Geometry: final body of the model. Coordinates: model frame, mm. Round coordinates to 2 decimals unless told otherwise and drop trailing zeros. Order: outer loops, then holes, each group sorted by start corner. A loop starts at its lowest first (then second) coordinate and runs counter-clockwise, first axis right, second up. Notation, with made-up numbers: (48, 39) -> (83, 39) arc R35 cw to (83, 78) -> close; hole circle Ø7 at (85, 47). An arc over 180 degrees is marked (long way). Put each result on its own line as item: value.
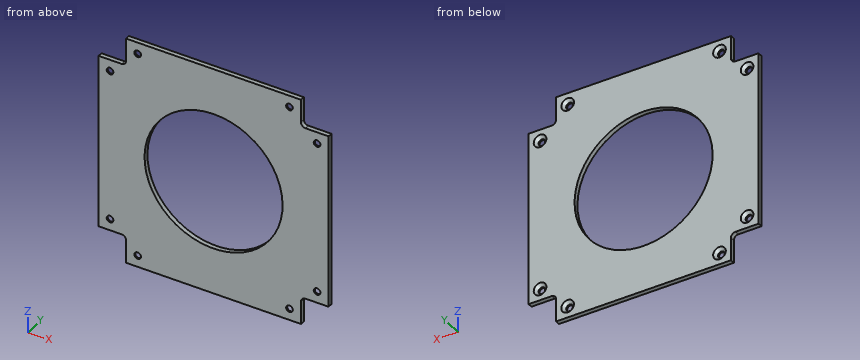
```python
from build123d import *

# Parameters (mm, degrees)
SCHIZZO1_R                              = 30
ESTRUSIONE_ESTRUSIONE1_DEPTH            = 1
RACCORDO1_R                             = 2
FORO_SVASATO_PER_VITE_M2_5_1_AT_2_COUNT = 2
FORO_SVASATO_PER_VITE_M2_5_1_AT_2_PITCH = 16.970562748
FORO_SVASATO_PER_VITE_M2_5_1_AT_3_COUNT = 2
FORO_SVASATO_PER_VITE_M2_5_1_AT_3_PITCH = 78.917678628
FORO_SVASATO_PER_VITE_M2_5_1_AT_4_COUNT = 2
FORO_SVASATO_PER_VITE_M2_5_1_AT_4_PITCH = 90
FORO_SVASATO_PER_VITE_M2_5_1_AT_5_COUNT = 2
FORO_SVASATO_PER_VITE_M2_5_1_AT_5_PITCH = 111.606451426
FORO_SVASATO_PER_VITE_M2_5_1_AT_6_COUNT = 2
FORO_SVASATO_PER_VITE_M2_5_1_AT_6_PITCH = 110.308657865
FORO_SVASATO_PER_VITE_M2_5_1_AT_7_COUNT = 2
FORO_SVASATO_PER_VITE_M2_5_1_AT_7_PITCH = 78.917678628
FORO_SVASATO_PER_VITE_M2_5_1_AT_8_COUNT = 2
FORO_SVASATO_PER_VITE_M2_5_1_AT_8_PITCH = 66


with BuildPart() as part:
    # Schizzo1 → Estrusione-Estrusione1 (new, symmetric)
    with BuildSketch(Plane(origin=(0, 0, 0), x_dir=(1, 0, 0), z_dir=(0, 1, 0))):
        Polygon((-50, -38), (-50, 38), (-38, 38), (-38, 50), (38, 50), (38, 38), (50, 38), (50, -38), (38, -38), (38, -50), (-38, -50), (-38, -38), align=None)
        with Locations(Location((0, 0, 0), (0, 0, 270))):
            Circle(SCHIZZO1_R, mode=Mode.SUBTRACT)
    extrude(amount=ESTRUSIONE_ESTRUSIONE1_DEPTH, both=True)

    # Raccordo1
    raccordo1_edges = [part.edges().sort_by_distance(p)[0] for p in [
        (-38, 0, -38),
        (38, 0, -38),
        (38, 0, 38),
        (-38, 0, 38),
    ]]
    fillet(raccordo1_edges, radius=RACCORDO1_R)

    # Schizzo4 → Foro svasato per Vite M2.5-1 (revolve, cut)
    with BuildSketch(Plane(origin=(-33, 1, -45), x_dir=(0, 0, 1), z_dir=(1, 0, 0))):
        Polygon((0, 0), (0, 2), (1.45, 2), (1.45, 1.3), (2.75, 0), align=None)
    foro_svasato_per_vite_m2_5_1 = revolve(axis=Axis((-33, 7.35, -45), (0, -1, 0)), mode=Mode.SUBTRACT)

    # Foro svasato per Vite M2.5-1 at 2: Foro svasato per Vite M2.5-1 ×2
    with Locations(*[Vector(-0.7071067811865476, 0, 0.7071067811865476) * (i * FORO_SVASATO_PER_VITE_M2_5_1_AT_2_PITCH) for i in range(1, FORO_SVASATO_PER_VITE_M2_5_1_AT_2_COUNT)]):
        add(foro_svasato_per_vite_m2_5_1, mode=Mode.SUBTRACT)

    # Foro svasato per Vite M2.5-1 at 3: Foro svasato per Vite M2.5-1 ×2
    with Locations(*[Vector(-0.15205718425394116, 0, 0.9883716976506172) * (i * FORO_SVASATO_PER_VITE_M2_5_1_AT_3_PITCH) for i in range(1, FORO_SVASATO_PER_VITE_M2_5_1_AT_3_COUNT)]):
        add(foro_svasato_per_vite_m2_5_1, mode=Mode.SUBTRACT)

    # Foro svasato per Vite M2.5-1 at 4: Foro svasato per Vite M2.5-1 ×2
    with Locations(*[(0, 0, i * FORO_SVASATO_PER_VITE_M2_5_1_AT_4_PITCH) for i in range(1, FORO_SVASATO_PER_VITE_M2_5_1_AT_4_COUNT)]):
        add(foro_svasato_per_vite_m2_5_1, mode=Mode.SUBTRACT)

    # Foro svasato per Vite M2.5-1 at 5: Foro svasato per Vite M2.5-1 ×2
    with Locations(*[Vector(0.5913636636275174, 0, 0.8064049958557056) * (i * FORO_SVASATO_PER_VITE_M2_5_1_AT_5_PITCH) for i in range(1, FORO_SVASATO_PER_VITE_M2_5_1_AT_5_COUNT)]):
        add(foro_svasato_per_vite_m2_5_1, mode=Mode.SUBTRACT)

    # Foro svasato per Vite M2.5-1 at 6: Foro svasato per Vite M2.5-1 ×2
    with Locations(*[Vector(0.7071067811865476, 0, 0.7071067811865476) * (i * FORO_SVASATO_PER_VITE_M2_5_1_AT_6_PITCH) for i in range(1, FORO_SVASATO_PER_VITE_M2_5_1_AT_6_COUNT)]):
        add(foro_svasato_per_vite_m2_5_1, mode=Mode.SUBTRACT)

    # Foro svasato per Vite M2.5-1 at 7: Foro svasato per Vite M2.5-1 ×2
    with Locations(*[Vector(0.9883716976506172, 0, 0.1520571842539412) * (i * FORO_SVASATO_PER_VITE_M2_5_1_AT_7_PITCH) for i in range(1, FORO_SVASATO_PER_VITE_M2_5_1_AT_7_COUNT)]):
        add(foro_svasato_per_vite_m2_5_1, mode=Mode.SUBTRACT)

    # Foro svasato per Vite M2.5-1 at 8: Foro svasato per Vite M2.5-1 ×2
    with Locations(*[(i * FORO_SVASATO_PER_VITE_M2_5_1_AT_8_PITCH, 0, 0) for i in range(1, FORO_SVASATO_PER_VITE_M2_5_1_AT_8_COUNT)]):
        add(foro_svasato_per_vite_m2_5_1, mode=Mode.SUBTRACT)


solid = part.part
```
1. Cut plane B-B on z = 45. Return loops of the section in (x, y).
Ans:
outline: (-38, -1) -> (-34.45, -1) -> (-34.45, -0.3) -> (-35.75, 1) -> (-38, 1) -> close; (-31.55, -1) -> (31.55, -1) -> (31.55, -0.3) -> (30.25, 1) -> (-30.25, 1) -> (-31.55, -0.3) -> close; (34.45, -1) -> (38, -1) -> (38, 1) -> (35.75, 1) -> (34.45, -0.3) -> close
2. Cut plane D-D on x = -8. Return loops of the section in (y, z).
Ans:
outline: (-1, -50) -> (1, -50) -> (1, -28.91) -> (-1, -28.91) -> close; (-1, 28.91) -> (1, 28.91) -> (1, 50) -> (-1, 50) -> close
3. Contact query for flat-ended pins moving along their axis: P1, Ø1.7, axis at x = 33, z = 45, coming from the -Y side; P2, Ø1, axis at x = 47.5, y = 0, coming from the -Z side; P3, Ø0.6, axis at y = 0.5, z = -44.5, coming from the +X side; P4, Ø3.5, axis at x = -33, z = -45, coming from the +Y side. Output: stop coordinate, or through.
Ans:
P1: through
P2: z = -38
P3: x = 38
P4: y = 0
4. Cut plane A-A on x = 45. Return loops of the section in (y, z).
Ans:
outline: (-1, -38) -> (1, -38) -> (1, -35.75) -> (-0.3, -34.45) -> (-1, -34.45) -> close; (-1, -31.55) -> (-0.3, -31.55) -> (1, -30.25) -> (1, 30.25) -> (-0.3, 31.55) -> (-1, 31.55) -> close; (-1, 34.45) -> (-0.3, 34.45) -> (1, 35.75) -> (1, 38) -> (-1, 38) -> close
5. Material intervals for probe 1 along Z at (x, y) = (-33, -0.5); probe 2 along X at (y, z) = (-0.5, 45); probe 3 along Z at (x, y) = (45.5, 0.7), sorted ascending.
Ans:
probe 1: -50 to -46.45, -43.55 to 43.55, 46.45 to 50
probe 2: -38 to -34.45, -31.55 to 31.55, 34.45 to 38
probe 3: -38 to -35.4, -30.6 to 30.6, 35.4 to 38
6. Cut plane C-C on y = 0.35. State how many separate pieces and enclosed holes the cut face has, and give its area (3 significant figures).
Ans:
separate pieces: 1
enclosed holes: 9
area: 6,490 mm²
